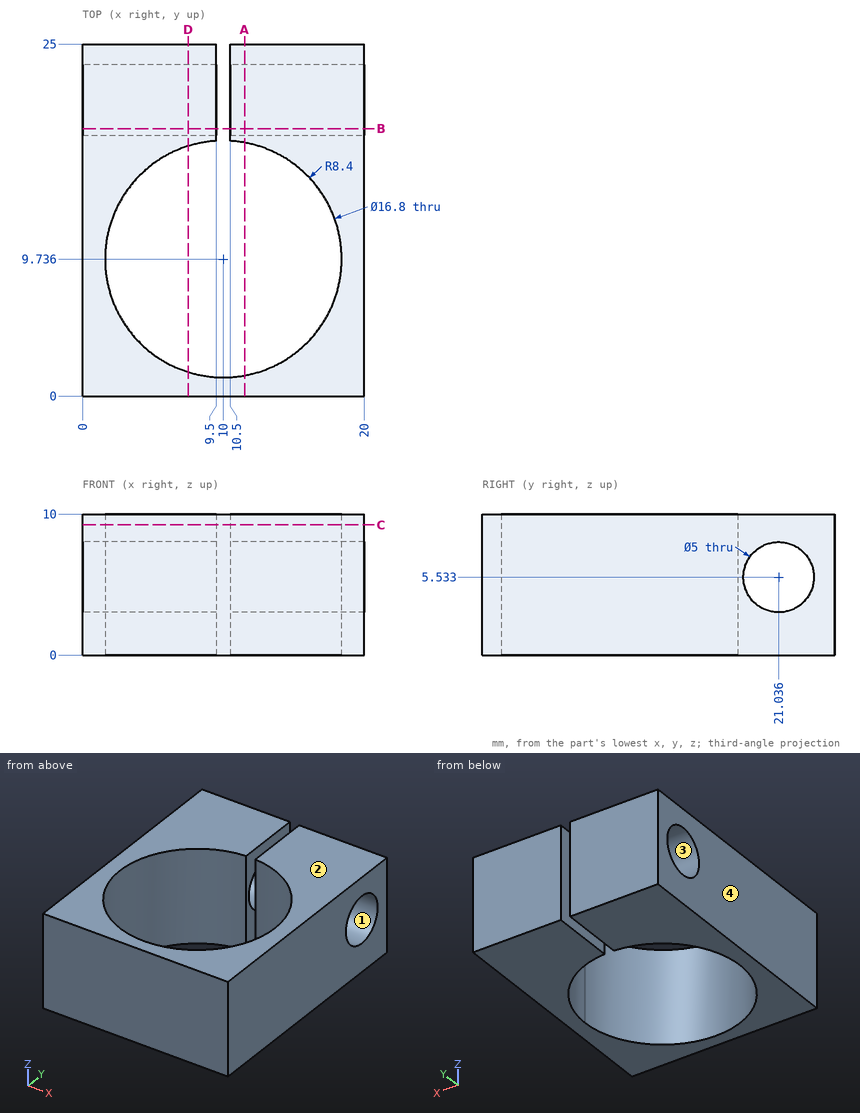
The figure shows three views and two pictorial views of one solid part (mm, origin at its lowest corner). Answer the questions. Give positions to 0.01 mm unless a question says otherwise; leave off trailing zeros. Loops run counter-clockwise (first coordinate to the right, second up) from the corner with the lowest first, then second, coordinate; pieces in that order, holes last. Notation, with made-up numbers: (47, 66.5) - (79, 66.5) arc R21 cw to (79, 77.5) - close; hole circle Ø6 at (-0.75, -17). An arc over 180 degrees is marked (long way). Use one line per item in the form item = value.
1. Section D-D on x = 7.5 is taken. Give the vertices of the cut face in (y, z) (1 decimal).
Calculated:
outline = (0, 0) - (1.7, 0) - (1.7, 10) - (0, 10) - close; (17.8, 0) - (25, 0) - (25, 10) - (17.8, 10) - close; hole circle Ø5 at (21, 5.5)
2. Section A-A on x = 11.5 is taken. Give the vertices of the cut face in (y, z) (1 decimal).
Calculated:
outline = (0, 0) - (1.5, 0) - (1.5, 10) - (0, 10) - close; (18, 0) - (25, 0) - (25, 10) - (18, 10) - close; hole circle Ø5 at (21, 5.5)
3. Section C-C on z = 9.25 is taken. Give the vertices of the cut face in (x, y) (1 decimal).
Calculated:
outline = (0, 0) - (20, 0) - (20, 25) - (10.5, 25) - (10.5, 18.1) arc R8.4 cw (long way) to (9.5, 18.1) - (9.5, 25) - (0, 25) - close
4. The mould has two halves that part along Z. Classify the marked faces 1, 2, 3 and 4: pulls with the +Z half, pulls with the -Z half, needs draft (parallel to the pull), parting line crosses it, or undercut.
Calculated:
face_1 = undercut
face_2 = pulls with the +Z half
face_3 = undercut
face_4 = needs draft
5. Given pin 1 Ø3 at (y, z) = (21.04, 5.53) entering from -X, flat-ended and moving along its own axis, determine where the tip first touches the part or whether it passes through.
Calculated:
pin_1 = through
6. Section B-B on y = 19 is taken. Give the vertices of the cut face in (x, z), then the cut area to 3 significant figures.
Calculated:
outline = (0, 0) - (9.5, 0) - (9.5, 4.08) - (0, 4.08) - close; (0, 6.98) - (9.5, 6.98) - (9.5, 10) - (0, 10) - close; (10.5, 0) - (20, 0) - (20, 4.08) - (10.5, 4.08) - close; (10.5, 6.98) - (20, 6.98) - (20, 10) - (10.5, 10) - close
area = 135 mm^2
7. Find the intervals of material crossed by line 1 along X through (y, z) = (9.5, 3); line 2 along X through (y, z) = (22.25, 2); line 3 along Y through (x, z) = (8.25, 7.25), in increasing order. Write a range as [from, to].
Calculated:
line_1 = [0, 1.6], [18.4, 20]
line_2 = [0, 9.5], [10.5, 20]
line_3 = [0, 1.52], [17.95, 19.22], [22.85, 25]
